Autodesk Inventor part; units mm, degrees
ref_plane "YZ Plane" through (0, 0, 0) normal (1, 0, 0) x (0, 1, 0)
ref_plane "XZ Plane" through (0, 0, 0) normal (0, 1, 0) x (-1, 0, 0)
ref_plane "XY Plane" through (0, 0, 0) normal (0, 0, 1) x (1, 0, 0)
sketch "Sketch1" plane through (0, 0, 0) normal (0, 1, 0) x (-1, 0, 0)
  line L0 (44.45, 127) -> (-44.45, 127)
  line L1 (-44.45, 127) -> (-44.45, -127)
  line L2 (-44.45, -127) -> (44.45, -127)
  line L3 (44.45, -127) -> (44.45, 127)
  point P0 (0, 0)
  dimension "d0" = 88.9
  dimension "d1" = 254
extrude "Extrusion1" add sketch "Sketch1" along normal blind 3.175
sketch "Sketch3" plane through (0, 3.175, 0) normal (0, 1, 0) x (1, 0, 0)
  line L0 (50.8, -114.3) -> (44.45, -114.3)
  line L1 (44.45, -114.3) -> (44.45, -88.9)
  line L2 (44.45, -88.9) -> (50.8, -88.9)
  line L3 (50.8, -88.9) -> (50.8, -114.3)
  line L4 (50.8, -63.5) -> (44.45, -63.5)
  line L5 (44.45, -63.5) -> (44.45, -38.1)
  line L6 (44.45, -38.1) -> (50.8, -38.1)
  line L7 (50.8, -38.1) -> (50.8, -63.5)
  line L8 (50.8, -12.7) -> (44.45, -12.7)
  line L9 (44.45, -12.7) -> (44.45, 12.7)
  line L10 (44.45, 12.7) -> (50.8, 12.7)
  line L11 (50.8, 12.7) -> (50.8, -12.7)
  line L12 (50.8, 38.1) -> (44.45, 38.1)
  line L13 (44.45, 38.1) -> (44.45, 63.5)
  line L14 (44.45, 63.5) -> (50.8, 63.5)
  line L15 (50.8, 63.5) -> (50.8, 38.1)
  line L16 (50.8, 88.9) -> (44.45, 88.9)
  line L17 (44.45, 88.9) -> (44.45, 114.3)
  line L18 (44.45, 114.3) -> (50.8, 114.3)
  line L19 (50.8, 114.3) -> (50.8, 88.9)
  point P0 (0, 0)
  dimension "d6" = 50.8
extrude "Extrusion2" add sketch "Sketch3" against normal blind 3.175
sketch "Sketch4" plane through (44.042, 3.175, 128.8813) normal (0, 1, 0) x (0, 0, -1)
  line L0 (8.2401, 85.8951) -> (239.8135, 85.8951) construction
  line L1 (239.8135, 85.8951) -> (239.8135, 3.5919) construction
  line L2 (239.8135, 3.5919) -> (8.2401, 3.5919) construction
  line L3 (8.2401, 3.5919) -> (8.2401, 85.8951) construction
  line L4 (47.8214, 10.1099) -> (33.1858, 10.1099)
  line L5 (33.1858, 10.1099) -> (33.1858, 61.3049)
  line L6 (33.1858, 61.3049) -> (15.4097, 61.3049)
  line L7 (15.4097, 61.3049) -> (15.4097, 70.8447)
  spline S0 degree 2 poles (15.4097, 70.8447) (25.9569, 71.9112) (30.4601, 74.2221) knots 0 0 0 1 1 1
  spline S1 degree 2 poles (30.4601, 74.2221) (35.6744, 77.007) (38.5186, 84.236) knots 0 0 0 1 1 1
  line L8 (38.5186, 84.236) -> (47.8214, 84.236)
  line L9 (47.8214, 84.236) -> (47.8214, 10.1099)
  spline S2 degree 2 poles (121.5327, 73.0371) (102.9271, 49.8689) (98.0091, 30.1968) knots 0 0 0 1 1 1
  spline S3 degree 2 poles (98.0091, 30.1968) (96.0537, 22.2568) (94.8687, 10.1099) knots 0 0 0 1 1 1
  line L10 (94.8687, 10.1099) -> (79.9368, 10.1099)
  spline S4 degree 2 poles (79.9368, 10.1099) (83.7883, 33.1002) (93.0911, 54.1352) (105.9491, 71.0817) knots 0 0 0 1 2 2 2
  line L11 (105.9491, 71.0817) -> (69.3897, 71.0817)
  line L12 (69.3897, 71.0817) -> (69.3897, 84.236)
  line L13 (69.3897, 84.236) -> (121.5327, 84.236)
  line L14 (121.5327, 84.236) -> (121.5327, 73.0371)
  spline S5 degree 2 poles (178.5939, 31.3226) (178.5939, 20.4792) (164.373, 7.6212) (152.4631, 7.6212) knots 0 0 0 1 2 2 2
  spline S6 degree 2 poles (152.4631, 7.6212) (142.5085, 7.6212) (135.8128, 12.8355) knots 0 0 0 1 1 1
  spline S7 degree 2 poles (135.8128, 12.8355) (127.5766, 19.2941) (127.5766, 31.8559) knots 0 0 0 1 1 1
  line L15 (127.5766, 31.8559) -> (141.7974, 31.8559)
  spline S8 degree 2 poles (141.7974, 31.8559) (141.2642, 25.3973) (145.5897, 21.9605) knots 0 0 0 1 1 1
  spline S9 degree 2 poles (145.5897, 21.9605) (148.9079, 19.2349) (153.7074, 19.2349) knots 0 0 0 1 1 1
  spline S10 degree 2 poles (153.7074, 19.2349) (157.6181, 19.2349) (163.7805, 27.2934) (163.7805, 31.7966) knots 0 0 0 1 2 2 2
  spline S11 degree 2 poles (163.7805, 31.7966) (163.7805, 37.485) (154.8925, 43.7066) (147.2488, 43.3511) knots 0 0 0 1 2 2 2
  line L16 (147.2488, 43.3511) -> (147.2488, 53.3057)
  spline S12 degree 2 poles (147.2488, 53.3057) (162.0621, 52.8909) (162.0621, 64.5638) knots 0 0 0 1 1 1
  spline S13 degree 2 poles (162.0621, 64.5638) (162.0621, 74.2814) (151.8113, 74.2814) knots 0 0 0 1 1 1
  spline S14 degree 2 poles (151.8113, 74.2814) (147.2488, 74.2814) (145.1156, 71.9705) knots 0 0 0 1 1 1
  spline S15 degree 2 poles (145.1156, 71.9705) (142.39, 68.9486) (142.0937, 60.8901) knots 0 0 0 1 1 1
  line L17 (142.0937, 60.8901) -> (128.7024, 60.8901)
  spline S16 degree 2 poles (128.7024, 60.8901) (128.5247, 62.5492) (128.5247, 64.149) knots 0 0 0 1 1 1
  spline S17 degree 2 poles (128.5247, 64.149) (128.5247, 73.7481) (142.2122, 85.8951) (152.6408, 85.8951) knots 0 0 0 1 2 2 2
  spline S18 degree 2 poles (152.6408, 85.8951) (163.1287, 85.8951) (169.3503, 80.977) knots 0 0 0 1 1 1
  spline S19 degree 2 poles (169.3503, 80.977) (176.1645, 75.7627) (176.1645, 66.0452) knots 0 0 0 1 1 1
  spline S20 degree 2 poles (176.1645, 66.0452) (176.1645, 60.4161) (174.2684, 56.9201) knots 0 0 0 1 1 1
  spline S21 degree 2 poles (174.2684, 56.9201) (172.7278, 54.2537) (168.0467, 49.8689) knots 0 0 0 1 1 1
  spline S22 degree 2 poles (168.0467, 49.8689) (178.5939, 43.0548) (178.5939, 31.3226) knots 0 0 0 1 1 1
  spline S23 degree 2 poles (236.7808, 34.7001) (236.7808, 22.8494) (230.0852, 15.3242) knots 0 0 0 1 1 1
  spline S24 degree 2 poles (230.0852, 15.3242) (223.0932, 7.6212) (211.4796, 7.6212) knots 0 0 0 1 1 1
  spline S25 degree 2 poles (211.4796, 7.6212) (195.4811, 7.6212) (189.7335, 22.4346) knots 0 0 0 1 1 1
  spline S26 degree 2 poles (189.7335, 22.4346) (186.0006, 32.0929) (186.0006, 51.4095) knots 0 0 0 1 1 1
  spline S27 degree 2 poles (186.0006, 51.4095) (186.0006, 66.2229) (192.874, 75.7627) knots 0 0 0 1 1 1
  spline S28 degree 2 poles (192.874, 75.7627) (200.2214, 85.8951) (212.7831, 85.8951) knots 0 0 0 1 1 1
  spline S29 degree 2 poles (212.7831, 85.8951) (222.56, 85.8951) (234.9439, 75.9997) (235.5365, 67.408) knots 0 0 0 1 2 2 2
  line L18 (235.5365, 67.408) -> (222.0859, 67.408)
  spline S30 degree 2 poles (222.0859, 67.408) (219.538, 74.1629) (212.1313, 74.1629) knots 0 0 0 1 1 1
  spline S31 degree 2 poles (212.1313, 74.1629) (206.7985, 74.1629) (200.2214, 65.5119) (200.2214, 58.52) knots 0 0 0 1 2 2 2
  spline S32 degree 2 poles (200.2214, 58.52) (200.2214, 56.0906) (200.6362, 53.4834) knots 0 0 0 1 1 1
  spline S33 degree 2 poles (200.6362, 53.4834) (207.3318, 59.231) (213.4942, 59.231) knots 0 0 0 1 1 1
  spline S34 degree 2 poles (213.4942, 59.231) (224.3376, 59.231) (236.7808, 46.6693) (236.7808, 34.7001) knots 0 0 0 1 2 2 2
  spline S35 degree 2 poles (222.9747, 35.1148) (222.9747, 41.1587) (217.2864, 47.8543) (212.3091, 47.8543) knots 0 0 0 1 2 2 2
  spline S36 degree 2 poles (212.3091, 47.8543) (207.1541, 47.8543) (200.2214, 39.7959) (200.2214, 33.1002) knots 0 0 0 1 2 2 2
  spline S37 degree 2 poles (200.2214, 33.1002) (200.2214, 27.5896) (206.5023, 19.9459) (211.1833, 19.9459) knots 0 0 0 1 2 2 2
  spline S38 degree 2 poles (211.1833, 19.9459) (216.5754, 19.9459) (222.9747, 28.3007) (222.9747, 35.1148) knots 0 0 0 1 2 2 2
  point P0 (127, 0)
extrude "Extrusion3" cut sketch "Sketch4" against normal blind 1.905
chamfer "Chamfer1" distance 3.175 angle 45 2 edges at (0, 0, 127) (0, 0, -127)
properties part number "side"
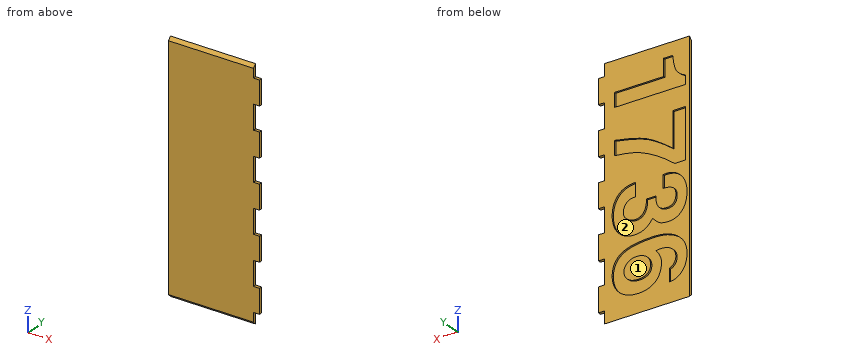
Geometry check sheet. Reference: the model listing, model coordinates, mm. Face numbers are marked on the shaded views. Round coordinates to 2 decimals unless told otherwise and drop trailing zeros. Write each loop counter-clockwise with the first axis right and the second up, starting at its lowest first coordinate (ties: lowest second). Pieces come first, ordered by that corner, then holes. Notation, with made-up numbers: (-18.5, 86) - (-0.5, 86) arc R30 ccw to (-0.5, 119) - close; hole circle Ø7 at (40, 65.25). An arc over 180 degrees is marked (long way). One line per item, written item: value.
1. Depth check by flat-ended pin: pin 1 Ø1.6 at (x, y) = (46.5, 2.5) entering from +Z; pin 2 Ø1.5 at (x, y) = (18.5, 2) entering from -Z; pin 3 Ø0.6 at (x, y) = (-18.5, 2.5) entering from +Z. Enter the tip coordinate at first touch or a pass-through.
The answers:
pin 1: stops at z = 114.3
pin 2: stops at z = -126.58
pin 3: stops at z = 126.63
2. Mould release check, pull along Z, two halves, no side actions. Record for the marked faces 1 and 2: released by +Z, released by -Z, zero draft, split by the parting line, or undercut.
The answers:
face 1: zero draft
face 2: undercut
3. Cross-section at A-A on z = 85.5. Record the boundary of the cut face in (x, y) (3 decimals).
The answers:
outline: (-44.45, 0) - (44.45, 0) - (44.45, 3.175) - (33.932, 3.175) - (33.932, 1.27) - (-40.194, 1.27) - (-40.194, 3.175) - (-44.45, 3.175) - close
4. Scan lines: L1, parallel to Z at x = -5, y = 1.3; L2, parallel to Z at x = 34, y = 2.9; L3, parallel to Y at x = -8, z = -29. Record each from-to range of solid material in increasing order.
The answers:
L1: z = -125.13 to -104.64, -57.13 to -40.38, -18.37 to 23.45, 37.73 to 81.06, 95.7 to 125.13
L2: z = -126.73 to -94.17, -71.34 to -36.39, -11.53 to 126.73
L3: y = 0 to 1.27
5. Cross-section at B-B on y = 1.8. Give the number of separate pieces and of enclosed holes in the cut face, and give its area (3 significant figures).
The answers:
separate pieces: 2
enclosed holes: 4
area: 15,900 mm^2
